from build123d import *

# Parameters (mm, degrees)
ENL_V_MAT_EXTRU_1_DEPTH = 1.5


with BuildPart() as part:
    # Esquisse1 → Base-Révolution (revolve)
    with BuildSketch(Plane.XY):
        with BuildLine():
            Line((0, 0), (1.25, 0))
            Line((1.25, 0), (1.5, 0.25))
            Line((1.5, 0.25), (1.5, 8.5))
            Line((1.5, 8.5), (5.5, 8.5))
            Line((5.5, 8.5), (5.5, 10))
            Line((5.5, 10), (3.926776695, 11.573223305))
            ThreePointArc((3.926776695, 11.573223305), (3.654329142, 11.627416493), (3.5, 11.396446609))
            Line((3.5, 11.396446609), (3.5, 10.5))
            Line((3.5, 10.5), (0, 10.5))
            Line((0, 10.5), (0, 0))
        make_face()
    revolve(axis=Axis((0, -3.120322121, 0), (0, 1, 0)))

    # Esquisse2 → Enlèv. mat.-Extru.1 (cut)
    with BuildSketch(Plane(origin=(0, 10.5, 0), x_dir=(-1, 0, 0), z_dir=(0, 1, 0))):
        Polygon((-0.649519053, 1.125), (0.649519053, 1.125), (1.299038106, 0), (0.649519053, -1.125), (-0.649519053, -1.125), (-1.299038106, 0), align=None)
    extrude(amount=-ENL_V_MAT_EXTRU_1_DEPTH, mode=Mode.SUBTRACT)


solid = part.part
Can you work these out from the model? Positions are in its coordinate system, mm. A direction names the side the tool comes from. Coordinates: 2 decimals unless noted, no trailing zeros. Write each loop counter-clockwise with the first axis right and the second up, starting at its lowest first coordinate (ties: lowest second). Pieces come first, ordered by that corner, then holes. Notation, with made-up numbers: (-28, 50) -> (12, 50) arc R19 ccw to (12, 83) -> close; hole circle Ø5 at (70, 83). An arc over 180 degrees is marked (long way). Answer as CSV lines item,"result".
1) If I drill on line 1 (Y direction, x = 3.25, z = -0.75); line 2 (X direction, y = 4, z = -0.75); line 3 (Z direction, x = 0, y = 11.25), over which ranges is the centre line in solid material (lowest first)? Write a range as from..to.
Check result:
line 1,"8.5..10.5"
line 2,"-1.3..1.3"
line 3,"-4.25..-3.5, 3.5..4.25"
2) On a 3-axis mill with a long thin cutter (end or side, diameter ignored), from which of +Z, -Z, +X, -X, +Y, -Y can I reach the whole of each face in a straight line? I mean faces 4 (the flat face through (0, 0, 0)), 5 (the cylindrical face through (-1.5, 4.43, -0.07)), 6 (the flat face through (0.98, 9.76, 0.55)). Say none if no direction works.
Check result:
face 4,"+Z, -Z, +X, -X, -Y"
face 5,"-Y"
face 6,"+Y"
3) Will these pins go through, and if not, where does the flat tip stop? P1, Ø2, axis at y = 6, z = 1.5, coming from the -X side; P2, Ø1.8, axis at x = 0, z = 0.5, coming from the +Y side.
Check result:
P1,"x = -1.41"
P2,"y = 10.5"
4) If we mould it in two halves opening along Z, with no side actions, what happens to faces 1 (the flat face through (0, 10, -1.125)), 2 (the cylindrical face through (-1.19, 9.26, 5.37)), 3 (the flat face through (1.3, 8.5, 1.1))? For each: +Z half, -Z half, draft (parallel to the pull), parting line (faces both ways), or undercut.
Check result:
face 1,"undercut"
face 2,"parting line"
face 3,"draft"
5) If we section it at B-B on y = 4: Please give me the cut outline in (x, z), then the cut area to 3 significant figures.
Check result:
outline,"circle Ø3 at (0, 0)"
area,"7.07 mm²"
6) If we section it at A-A on x = 0: Please give me the cut outline in (y, z) (3 decimals).
Check result:
outline,"(0, -1.25) -> (0.25, -1.5) -> (8.5, -1.5) -> (8.5, -5.5) -> (10, -5.5) -> (11.573, -3.927) arc R0.25 ccw to (11.396, -3.5) -> (10.5, -3.5) -> (10.5, -1.125) -> (9, -1.125) -> (9, 1.125) -> (10.5, 1.125) -> (10.5, 3.5) -> (11.396, 3.5) arc R0.25 ccw to (11.573, 3.927) -> (10, 5.5) -> (8.5, 5.5) -> (8.5, 1.5) -> (0.25, 1.5) -> (0, 1.25) -> close"
